Model file for the job. Use its own axes, mm. Face numbers are marked on the shaded views. Coordinates: 2 decimals unless noted, no trailing zeros. Loops run counter-clockwise (first coordinate to the right, second up) from the corner with the lowest first, then second, coordinate; pieces in that order, holes last. Notation, with made-up numbers: (-10.5, 2.25) -> (7.5, 2.25) arc R22 cw to (7.5, 28.25) -> close; hole circle Ø10 at (76, -13). An arc over 180 degrees is marked (long way). Use one line per item in the form item = value.
```python
from build123d import *

# Parameters (mm, degrees)
SKETCH1_W                                  = 16
SKETCH1_H                                  = 16
BASE_DEPTH                                 = 50
SKETCH2_R                                  = 5
RODSLOT_DEPTH                              = 54.103672189
RODSCREWMOUNT_REACH                        = 55.104
SKETCH3_R                                  = 2.55
CHAMFERFORRODSCREW_SIZE                    = 0.5
M5X0_8_TAPPED_HOLE_FOR_ROD_SCREW_D         = 4.2
M5X0_8_TAPPED_HOLE_FOR_ROD_SCREW_DEPTH     = 7.6381927
M5X0_8_TAPPED_HOLE_FOR_ROD_SCREW_TIP       = 1.2618073
M3X0_5_TAPPED_HOLE_FOR_MOUNT_WITH_SECOND_D = 2.5


with BuildPart() as part:
    # Sketch1 → Base (new body)
    with BuildSketch(Plane.XY):
        Rectangle(SKETCH1_W, SKETCH1_H)
    extrude(amount=BASE_DEPTH)

    # Sketch2 → RodSlot (cut, through all)
    with BuildSketch(Plane(origin=(0, 8, 0), x_dir=(1, 0, 0), z_dir=(0, 1, 0))):
        with Locations((0, -30)):
            Circle(SKETCH2_R)
        with BuildLine():
            Line((-1, -34.898979486), (-1, -50))
            Line((-1, -50), (1, -50))
            Line((1, -50), (1, -34.898979486))
            ThreePointArc((1, -34.898979486), (0, -35), (-1, -34.898979486))
        make_face()
    extrude(amount=-RODSLOT_DEPTH, mode=Mode.SUBTRACT)

    # Sketch3 → RodScrewMount (cut, up to next)
    with BuildSketch(Plane(origin=(8, 0, 0), x_dir=(0, 0, -1), z_dir=(1, 0, 0)), mode=Mode.PRIVATE) as rodscrewmount_sk1:
        with Locations((-45, 0)):
            Circle(SKETCH3_R)
    rodscrewmount_tool1 = extrude(rodscrewmount_sk1.sketch, amount=-RODSCREWMOUNT_REACH, mode=Mode.PRIVATE) & part.part
    add(rodscrewmount_tool1.solids().sort_by_distance((8, 0, 45))[0], mode=Mode.SUBTRACT)

    # ChamferForRodScrew
    chamferforrodscrew_edges = [part.edges().sort_by_distance(p)[0] for p in [
        (8, 0, 47.55),
    ]]
    chamfer(chamferforrodscrew_edges, length=CHAMFERFORRODSCREW_SIZE)

    # M5x0.8 Tapped Hole for rod screw
    with Locations(Plane.ZY.offset(8)):
        with Locations((45, 0)):
            Hole(M5X0_8_TAPPED_HOLE_FOR_ROD_SCREW_D / 2, depth=M5X0_8_TAPPED_HOLE_FOR_ROD_SCREW_DEPTH)
            with Locations((0, 0, -(M5X0_8_TAPPED_HOLE_FOR_ROD_SCREW_DEPTH + M5X0_8_TAPPED_HOLE_FOR_ROD_SCREW_TIP / 2))):  # 118° drill point
                Cone(0, M5X0_8_TAPPED_HOLE_FOR_ROD_SCREW_D / 2, M5X0_8_TAPPED_HOLE_FOR_ROD_SCREW_TIP, mode=Mode.SUBTRACT)

    # M3x0.5 Tapped Hole for mount with second part (through all)
    with Locations(Plane.ZY.offset(8)):
        with Locations((5, 3), (11, -3)):
            Hole(M3X0_5_TAPPED_HOLE_FOR_MOUNT_WITH_SECOND_D / 2)


solid = part.part
```
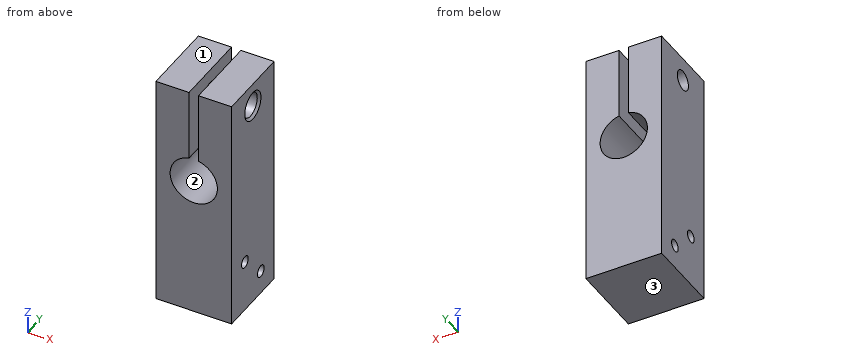
Q1. Mould opens along Z. For the marked faces 1, 2 and 3 say: released by +Z, released by -Z, zero draft, split by the parting line, or undercut.
Result:
face_1 = released by +Z
face_2 = undercut
face_3 = released by -Z
Q2. Band-saw the part on D-D, the plane y = 6. Write the cut outline in (x, z), and give its area (3 significant figures).
Result:
outline = (-8, 0) -> (8, 0) -> (8, 50) -> (1, 50) -> (1, 34.9) arc R5 cw (long way) to (-1, 34.9) -> (-1, 50) -> (-8, 50) -> close
area = 691 mm2
Q3. Wall check: line 1 along Y through (x, z) = (-1.25, 5); line 2 along Z through (x, y) = (3.75, -1.5); line 3 along Z through (x, y) = (4.25, -0.5). Give the ranges that are in metal, low to high.
Result:
line_1 = -8 to 1.75, 4.25 to 8
line_2 = 0 to 26.69, 33.31 to 42.94, 47.06 to 50
line_3 = 0 to 27.37, 32.63 to 42.5, 47.5 to 50
Q4. Band-saw the part on B-B, the plane x = 4. Write the cut outline in (y, z), and give its area (3 significant figures).
Result:
outline = (-8, 0) -> (8, 0) -> (8, 27) -> (-8, 27) -> close; (-8, 33) -> (8, 33) -> (8, 50) -> (-8, 50) -> close; hole circle Ø2.5 at (-3, 11); hole circle Ø5.1 at (0, 45); hole circle Ø2.5 at (3, 5)
area = 674 mm2
Q5. Band-saw the part on A-A, the plane z = 45. Write the cut outline in (x, y), and give its area (3 significant figures).
Result:
outline = (-8, -8) -> (-1, -8) -> (-1, -2.1) -> (-8, -2.1) -> close; (-8, 2.1) -> (-1, 2.1) -> (-1, 8) -> (-8, 8) -> close; (1, -8) -> (8, -8) -> (8, -3.05) -> (7.5, -2.55) -> (1, -2.55) -> close; (1, 2.55) -> (7.5, 2.55) -> (8, 3.05) -> (8, 8) -> (1, 8) -> close
area = 159 mm2
Q6. Pin check, flat tips, straight feed: pin 1 Ø5.5 at (y, z) = (0, 45) entering from +X; pin 2 Ø4.5 at (y, z) = (0, 45) entering from +X. Stop position of each tip, or through.
Result:
pin_1 = 7.7
pin_2 = -1
Q7. Band-saw the part on C-C, the plane z = 11. Write the cut outline in (x, y), and give its area (3 significant figures).
Result:
outline = (-8, -8) -> (8, -8) -> (8, -4.25) -> (-8, -4.25) -> close; (-8, -1.75) -> (8, -1.75) -> (8, 8) -> (-8, 8) -> close
area = 216 mm2
